Could you check a few things on this model? Use its own coordinates, in mm. A direction names the side the tool comes from. Coordinates: 2 decimals unless noted, no trailing zeros. Write each loop counter-clockwise with the first axis right and the second up, starting at its lowest first coordinate (ties: lowest second). Pieces come first, ordered by that corner, then holes. Notation, with made-up numbers: M 16,-10.75 L 39,-10.75 A22 cw 39,5.25 Z; hole C 75,82 d5. An arc over 180 degrees is marked long. Answer as CSV lines item,"result". Start each with the question number.
Item 1: If I drill on line 1 along Y through (x, z) = (-2, -18); line 2 along X through (y, z) = (3.5, 11.5); line 3 along Z through (x, y) = (-6.5, 18.5), over which ranges is the centre line in solid material (lowest first)? Write a range as [from, to].
Item 2: Suppose I cut it at A-A, the plane y = 17.75. Write out the boundary of the cut face in (x, z).
Item 3: On a 3-axis mill with a long thin cutter (end or side, diameter ignored), from which of +Z, -Z, +X, -X, +Y, -Y can I reach the whole of each face in a straight line? I mean faces 4 (the flat face through (-15, 9, 8)), 5 (the flat face through (0.21, 9.271, 5.856)), 6 (the flat face through (10.07, 17.75, 2.81)), 7 (the flat face through (15, 9, 8)), 8 (the cylindrical face through (31.44, 1.01, -19.12)). Say none if no direction works.
Item 4: Suppose I cut it at C-C, the plane z = 13. Write out the boundary of the cut face in (x, y).
Item 5: Suppose I cut it at D-D, the plane y = 7.25. Write out the boundary of the cut face in (x, z).
Item 6: I'm going to push flat-ended pins straight in: P1, Ø1, axis at x = -10, y = 16.5, coming from the +Z side; P2, Ø8, axis at x = -22.5, y = 6.5, coming from the +Z side; P3, Ø2, axis at y = 16, z = 3, coming from the -X side; P4, Ø1.5, axis at x = 8.5, y = 15, coming from the +Z side. Where does each tip first touch, or does it pass through?
Item 7: We'd pull the mould along Z, two halves only. Please class faces 1 (the flat face through (-9.93, 18.85, 5.42)), 2 (the cylindrical face through (10.07, 20.535, 4.74)), 3 (the cylindrical face through (-31.8, 0.99, -4.25)): +Z half, -Z half, draft (parallel to the pull), parting line (faces both ways), or undercut.
Item 8: Suppose I cut it at B-B, the plane x = 26.5. Write out the boundary of the cut face in (y, z), and give its area (3 significant figures).
```python
from build123d import *

# Parameters (mm, degrees)
BOSS_EXTRUDE2_DEPTH = 2
BOSS_EXTRUDE3_DEPTH = 15
CHAMFER1_SIZE       = 5
CHAMFER1_SIZE2      = 3.535533906
FILLET2_R           = 5
FILLET3_R           = 2
SKETCH6_R           = 5
CUT_EXTRUDE5_DEPTH  = 43.63874873
FILLET4_R           = 4
SKETCH4_R           = 4
CUT_EXTRUDE6_DEPTH  = 5


with BuildPart() as part:
    # Sketch1 → Boss-Extrude2 (new body)
    with BuildSketch(Plane(origin=(0, 0, 0), x_dir=(1, 0, 0), z_dir=(0, 1, 0))):
        with BuildLine():
            Line((-30.372025328, 4.851856012), (-20.222025328, 4.851856012))
            ThreePointArc((-20.222025328, 4.851856012), (-18.454258375, 5.584089059), (-17.722025328, 7.351856012))
            Line((-17.722025328, 7.351856012), (-17.722025328, 20.326643656))
            Line((-17.722025328, 20.326643656), (32.577974672, 20.326643656))
            Line((32.577974672, 20.326643656), (32.577974672, -18.198143988))
            ThreePointArc((32.577974672, -18.198143988), (31.992188234, -19.612357551), (30.577974672, -20.198143988))
            Line((30.577974672, -20.198143988), (-30.372025328, -20.198143988))
            ThreePointArc((-30.372025328, -20.198143988), (-31.78623889, -19.612357551), (-32.372025328, -18.198143988))
            Line((-32.372025328, -18.198143988), (-32.372025328, 2.851856012))
            ThreePointArc((-32.372025328, 2.851856012), (-31.78623889, 4.266069574), (-30.372025328, 4.851856012))
        make_face()
    extrude(amount=BOSS_EXTRUDE2_DEPTH)

    # Sketch2 → Boss-Extrude3 (add, symmetric)
    with BuildSketch(Plane(origin=(0, 0, 0), x_dir=(0, 0, -1), z_dir=(1, 0, 0))):
        with BuildLine():
            Line((-20.198143988, 2), (-8.198143988, 14))
            Line((-8.198143988, 14), (-8.198143988, 17))
            ThreePointArc((-8.198143988, 17), (-4.662610082, 20.535533906), (-1.127076177, 17))
            Line((-1.127076177, 17), (-1.127076177, 14))
            Line((-1.127076177, 14), (-13.127076177, 2))
            Line((-13.127076177, 2), (-20.198143988, 2))
        make_face()
        Polygon((-4.662610082, 14.835215599), (-3.131876353, 15.469266271), (-2.497825682, 17), (-3.131876353, 18.530733729), (-4.662610082, 19.164784401), (-6.193343812, 18.530733729), (-6.827394483, 17), (-6.193343812, 15.469266271), align=None, mode=Mode.SUBTRACT)
    extrude(amount=BOSS_EXTRUDE3_DEPTH, both=True)

    # Chamfer1
    chamfer1_edges = [part.edges().sort_by_distance(p)[0] for p in [
        (0, 2, 13.127076177),
    ]]
    chamfer1_side = [part.faces().sort_by_distance(p)[0] for p in [
        (2.715334419, 2, -0.404703372),
    ]]
    chamfer(chamfer1_edges, length=CHAMFER1_SIZE, length2=CHAMFER1_SIZE2, reference=chamfer1_side[0])

    # Fillet2
    fillet2_edges = [part.edges().sort_by_distance(p)[0] for p in [
        (0, 14, 1.127076177),
        (0, 14, 8.198143988),
    ]]
    fillet(fillet2_edges, radius=FILLET2_R)

    # Fillet3
    fillet3_edges = [part.edges().sort_by_distance(p)[0] for p in [
        (0, 4.5, 10.627076177),
    ]]
    fillet(fillet3_edges, radius=FILLET3_R)

    # Sketch6 → Cut-Extrude5 (cut, through all)
    with BuildSketch(Plane(origin=(0, 2, 0), x_dir=(1, 0, 0), z_dir=(0, 1, 0))):
        with Locations(Location((22.577974672, 10.326643656, 0), (0, 0, 270))):
            Circle(SKETCH6_R)
        with Locations(Location((-7.722025328, 10.326643656, 0), (0, 0, 270))):
            Circle(SKETCH6_R)
        with Locations(Location((-22.372025328, -5.148143988, 0), (0, 0, 270))):
            Circle(SKETCH6_R)
    extrude(amount=-CUT_EXTRUDE5_DEPTH, mode=Mode.SUBTRACT)

    # Fillet4
    fillet4_edges = [part.edges().sort_by_distance(p)[0] for p in [
        (-17.722025328, 1, -20.326643656),
        (32.577974672, 1, -20.326643656),
    ]]
    fillet(fillet4_edges, radius=FILLET4_R)

    # Sketch4 → Cut-Extrude6 (cut, symmetric)
    with BuildSketch(Plane(origin=(0, 0, 0), x_dir=(0, 0, -1), z_dir=(1, 0, 0))):
        with Locations((-4.662610082, 17)):
            Circle(SKETCH4_R)
    extrude(amount=CUT_EXTRUDE6_DEPTH, both=True, mode=Mode.SUBTRACT)

    # Chamfer2
    # the kernel refuses this chamfer: 1, 0.7919938 mm, written as the material it takes off along each edge
    with BuildSketch(Plane(origin=(-5, 14.878966184, 1.271265873), x_dir=(0, -0.9451293826533955, 0.3266962657350272), z_dir=(1, 0, 0))) as chamfer2_piece_1:
        with BuildLine():
            Line((0.919369635, 0), (0.720278223, -0.239594389))
            ThreePointArc((0.720278223, -0.239594389), (0.358867912, -0.100362012), (0, 0))
            ThreePointArc((0, 0), (0.472481659, 0.021159479), (0.919369635, 0))
        make_face()
    extrude(amount=10, mode=Mode.SUBTRACT)

    # Chamfer3
    # the kernel refuses this chamfer: 1, 0.717753161 mm, written as the material it takes off along each edge
    with BuildSketch(Plane(origin=(5, 15.260052087, 8.264357056), x_dir=(0, -0.8256881187536859, -0.5641268745140575), z_dir=(-1, 0, 0))) as chamfer3_piece_1:
        with BuildLine():
            Line((1.190375888, 0), (0.477865365, 0.526129749))
            ThreePointArc((0.477865365, 0.526129749), (0.246923946, 0.253056093), (0, 0))
            ThreePointArc((0, 0), (0.611506956, 0.044495651), (1.190375888, 0))
        make_face()
    extrude(amount=10, mode=Mode.SUBTRACT)


solid = part.part
```
Ans:
1,line 1,"y = [0, 2]"
1,line 2,"x = [-15, 15]"
1,line 3,"z = [1.46, 3.12], [6.21, 7.86]"
2,outline,"M -15,1.21 L -5,1.21 L -5,2.81 L -15,2.81 Z; M -15,6.52 L -5,6.52 L -5,8.12 L -15,8.12 Z; M 5,1.21 L 15,1.21 L 15,2.81 L 5,2.81 Z; M 5,6.52 L 15,6.52 L 15,8.12 L 5,8.12 Z"
3,face 4,"+Z, -Z, -X, +Y"
3,face 5,"-Z, +X, -X"
3,face 6,"+X, -X"
3,face 7,"+Z, -Z, +X, +Y"
3,face 8,"-Z, +X, +Y, -Y"
4,outline,"M -32.37,0 L 32.58,0 L 32.58,2 L 15,2 L 15,9.2 L -15,9.2 L -15,2 L -32.37,2 Z"
5,outline,"M -15,7.88 L 15,7.88 L 15,14.95 L -15,14.95 Z"
6,P1,"stops at z = 8.2"
6,P2,"passes through"
6,P3,"stops at x = -15"
6,P4,"stops at z = 8.54"
7,face 1,"undercut"
7,face 2,"parting line"
7,face 3,"-Z half"
8,outline,"M 0,-20.33 L 2,-20.33 L 2,-13.43 L 0,-13.43 Z; M 0,-7.23 L 2,-7.23 L 2,20.2 L 0,20.2 Z"
8,area,"68.6 mm^2"
